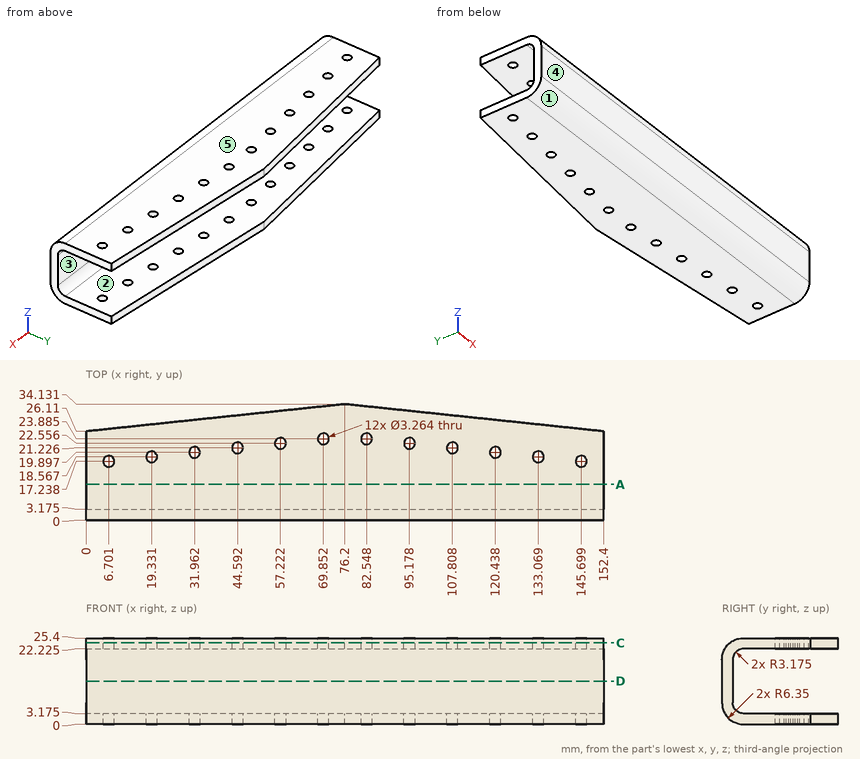
Input: dimensioned drawing with shaded views. Units: mm. Origin: part minimum x, y, z. A direction names the side the tool comes from. Round coordinates to 2 decimals unless told otherwise and drop trailing zeros. Order: outer loops, then holes, each group sorted by start corner. A loop starts at its lowest first (then second) coordinate and runs counter-clockwise, first axis right, second up.
Q1. Section C-C, the plane z = 24. Give the number of separate pieces and of enclosed holes in the cut face, and give its area (3 significant figures).
Result sheet:
separate pieces: 1
enclosed holes: 12
area: 4,130 mm2
Q2. Pin query (flat end, axial travel): pin 1 (4 mm diameter, centred on x = 31.96, y = 19.9, fed in from -Z); pin 2 (4 mm diameter, centred on x = 47, z = 10.5, fed in from +Y) (3 decimals). Return the tip coordinate at first contact, or that it passes through.
Result sheet:
pin 1: stops at z = 0
pin 2: stops at y = 3.175
Q3. Access query for the marked faces 1 and 2. Directions: +Z, -Z, +X, -X, +Y, -Y. A direction counts if a zero-diameter tool reaches every point of the face in a straight line with its end or side. Return the directions, or none.
Result sheet:
face 1: -Z, +X, -X, -Y
face 2: +X, -X, +Y
Q4. Section D-D, the plane z = 12.75. Output: boundary loops of the cut face in (x, y) (1 decimal).
Result sheet:
outline: (0, 0) - (152.4, 0) - (152.4, 3.2) - (0, 3.2) - close
Q5. Material intervals for probe 1 along Z at (x, y) = (34.5, 20) (1 decimal); probe 2 along Y at (x, z) = (44, 8.75) (1 decimal); probe 3 along X at (y, z) = (19, 24.75) (1 decimal), sorted ascending.
Result sheet:
probe 1: z = 0 to 3.2, 22.2 to 25.4
probe 2: y = 0 to 3.2
probe 3: x = 0 to 17.8, 20.9 to 30.6, 33.3 to 119.1, 121.8 to 131.5, 134.6 to 152.4
Q6. Mould query, pull axis Z, two halves, no side actions, for the marked faces 3, 4 and 5. Classes: released by +Z, released by -Z, zero draft, split by the parting line, or undercut.
Result sheet:
face 3: undercut
face 4: zero draft
face 5: released by +Z
Q7. Section A-A, the plane y = 10.5. Output: boundary loops of the cut face in (x, z) (1 decimal).
Result sheet:
outline: (0, 0) - (152.4, 0) - (152.4, 3.2) - (0, 3.2) - close; (0, 22.2) - (152.4, 22.2) - (152.4, 25.4) - (0, 25.4) - close
